Build history of the part. All positions in model axes, mm. A direction names the side the tool comes from. Round coordinates to 2 decimals unless told otherwise and drop trailing zeros. Order: outer loops, then holes, each group sorted by start corner. A loop starts at its lowest first (then second) coordinate and runs counter-clockwise, first axis right, second up. Notation, with made-up numbers: (64, 26) -> (89, 26) arc R20 cw to (89, 42) -> close; hole circle Ø11 at (-11.5, 87.5). An arc over 180 degrees is marked (long way). Answer as CSV lines item,"result". Start each with the question number.
```python
from build123d import *

# Parameters (mm, degrees)
BOSS_EXTRUDE1_DEPTH      = 7.5
SKETCH4_W                = 20
SKETCH4_H                = 3
BOSS_EXTRUDE2_DEPTH      = 35
SKETCH6_W                = 20
SKETCH6_H                = 3
BOSS_EXTRUDE3_DEPTH      = 59.4
SKETCH5_R                = 1.678965669
SKETCH5_R_2              = 1.417070449
SKETCH5_R_3              = 1.591812116
SKETCH5_R_4              = 1.461089302
CUT_EXTRUDE1_DEPTH       = 132.345384388
SKETCH7_R                = 1.6
CUT_EXTRUDE2_DEPTH       = 132.345384388
SKETCH10_W               = 33
SKETCH10_H               = 3
BOSS_EXTRUDE4_DEPTH      = 10
SKETCH11_W               = 8
SKETCH11_H               = 7.5
CUT_EXTRUDE4_DEPTH       = 133.017460966
SKETCH12_W               = 10
SKETCH12_H               = 3
BOSS_EXTRUDE5_DEPTH      = 10
CHAMFER1_SIZE            = 10
CHAMFER1_OF_MIRROR6_SIZE = 10
MIRROR7_START            = -40.25
MIRROR7_DEPTH            = 3
MIRROR7_START_2          = 2.25
MIRROR7_2_DEPTH          = 3
CUT_EXTRUDE5_DEPTH       = 132.345384388


# Read off the part's stored shape, not the designer's step: Mirror7
with BuildPart() as part:
    # Sketch3 → Boss-Extrude1 (new body)
    with BuildSketch(Plane.XY):
        Polygon((0, 0), (19.5, 0), (19.5, 28), (58.5, 28), (58.5, 0), (78, 0), (78, -3), (55.5, -3), (55.5, 25), (22.5, 25), (22.5, -3), (0, -3), align=None)
    boss_extrude1 = extrude(amount=BOSS_EXTRUDE1_DEPTH)

    # Sketch4 → Boss-Extrude2 (add)
    with BuildSketch(Plane(origin=(0, 0, 0), x_dir=(-1, 0, 0), z_dir=(0, 0, -1))):
        with Locations((-39, 26.5)):
            Rectangle(SKETCH4_W, SKETCH4_H)
    extrude(amount=BOSS_EXTRUDE2_DEPTH)

    # Mirror1: Boss-Extrude1 across plane
    add(boss_extrude1.mirror(Plane(origin=(0, 0, -17.5), x_dir=(1, 0, 0), z_dir=(0, 0, -1))))

    # Sketch6 → Boss-Extrude3 (add)
    with BuildSketch(Plane(origin=(0, 0, -42.5), x_dir=(-1, 0, 0), z_dir=(0, 0, -1))):
        with Locations((-39, 26.5)):
            Rectangle(SKETCH6_W, SKETCH6_H)
    extrude(amount=BOSS_EXTRUDE3_DEPTH)

    # Sketch5 → Cut-Extrude1 (cut, through all)
    with BuildSketch(Plane(origin=(0, 0, 0), x_dir=(1, 0, 0), z_dir=(0, 1, 0))):
        with Locations(Location((74, -3.75, 0), (0, 0, 270))):
            Circle(SKETCH5_R)
        with Locations(Location((4, -3.75, 0), (0, 0, 270))):
            Circle(SKETCH5_R_2)
        with Locations(Location((4, 38.75, 0), (0, 0, 270))):
            Circle(SKETCH5_R_3)
        with Locations(Location((74, 38.75, 0), (0, 0, 270))):
            Circle(SKETCH5_R_4)
    extrude(amount=-CUT_EXTRUDE1_DEPTH, mode=Mode.SUBTRACT)

    # Mirror5: Boss-Extrude1 across plane
    add(boss_extrude1.mirror(Plane(origin=(0, 0, -47.2), x_dir=(1, 0, 0), z_dir=(0, 0, -1))))

    # Sketch7 → Cut-Extrude2 (cut, through all)
    with BuildSketch(Plane(origin=(0, 0, 0), x_dir=(1, 0, 0), z_dir=(0, 1, 0))):
        with Locations(Location((64.4, 98.15, 0), (0, 0, 270))):
            Circle(SKETCH7_R)
        with Locations(Location((13.6, 98.15, 0), (0, 0, 270))):
            Circle(SKETCH7_R)
    extrude(amount=-CUT_EXTRUDE2_DEPTH, mode=Mode.SUBTRACT)

    # Sketch10 → Boss-Extrude4 (add)
    with BuildSketch(Plane.XZ.offset(-25)):
        with Locations((39, 6)):
            Rectangle(SKETCH10_W, SKETCH10_H)
    extrude(amount=BOSS_EXTRUDE4_DEPTH)

    # Sketch11 → Cut-Extrude4 (cut, through all)
    with BuildSketch(Plane.XZ.offset(3)):
        with Locations((4, -98.15)):
            Rectangle(SKETCH11_W, SKETCH11_H)
        with Locations((74, -98.15)):
            Rectangle(SKETCH11_W, SKETCH11_H)
    extrude(amount=-CUT_EXTRUDE4_DEPTH, mode=Mode.SUBTRACT)

    # Sketch12 → Boss-Extrude5 (add)
    with BuildSketch(Plane(origin=(0, 0, 0), x_dir=(1, 0, 0), z_dir=(0, 1, 0))):
        with Locations((14.5, 38.75)):
            Rectangle(SKETCH12_W, SKETCH12_H)
    boss_extrude5 = extrude(amount=BOSS_EXTRUDE5_DEPTH)

    # Chamfer1
    chamfer1_edges = [part.edges().sort_by_distance(p)[0] for p in [
        (9.5, 10, -38.75),
    ]]
    chamfer(chamfer1_edges, length=CHAMFER1_SIZE - 0.0001)  # a hair under: the kernel refuses the full size

    # Mirror6: Boss-Extrude5 across plane
    add(boss_extrude5.mirror(Plane.XY.offset(-17.5)))

    # Chamfer1 of Mirror6
    chamfer1_of_mirror6_edges = [part.edges().sort_by_distance(p)[0] for p in [
        (9.5, 10, 3.75),
    ]]
    chamfer(chamfer1_of_mirror6_edges, length=CHAMFER1_OF_MIRROR6_SIZE - 0.0001)  # a hair under: the kernel refuses the full size

    # Mirror7 outline → Mirror7 (add)
    with BuildSketch(Plane.XY.offset(MIRROR7_START)):
        Polygon((58.5, 0), (68.5, 0), (58.5, 10), align=None)
    extrude(amount=MIRROR7_DEPTH)

    # Mirror7 2 outline → Mirror7 2 (add)
    with BuildSketch(Plane.XY.offset(MIRROR7_START_2)):
        Polygon((58.5, 0), (68.5, 0), (58.5, 10), align=None)
    extrude(amount=MIRROR7_2_DEPTH)

    # Sketch13 → Cut-Extrude5 (cut, through all)
    with BuildSketch(Plane.XZ.offset(-25)):
        with BuildLine():
            Line((43, -5.187147638), (43, -27.972265557))
            ThreePointArc((43, -27.972265557), (39, -31.972265557), (35, -27.972265557))
            Line((35, -27.972265557), (35, -5.187147638))
            ThreePointArc((35, -5.187147638), (39, -1.187147638), (43, -5.187147638))
        make_face()
        with BuildLine():
            Line((43, -52.417226503), (43, -84.557823303))
            ThreePointArc((43, -84.557823303), (39, -88.557823303), (35, -84.557823303))
            Line((35, -84.557823303), (35, -52.417226503))
            ThreePointArc((35, -52.417226503), (39, -48.417226503), (43, -52.417226503))
        make_face()
    extrude(amount=-CUT_EXTRUDE5_DEPTH, mode=Mode.SUBTRACT)


solid = part.part
```
Q1. Slice it at B-B, the plane z = -18. Write the cut outline in (x, y).
Q2. Which spindle directions (+Z, -Z, +X, -X, +Y, -Y) get a long thin tool onto all of the face, cutting with end or side? Do faces 4 (the face through (58, 9, -42.5)), 5 (the face through (7, 0, 4)), 6 (the face through (16, 4, -40.25)), 7 (the face through (35, 26, -17)). Say none if no direction does.
Q3. Probe L1, parallel to Z at x = 20.5, y = 2; L2, parallel to X at y = -0.8, z = 3.75; L3, parallel to Z at x = 74, y = -1.3. List the from-to ranges inside material, lowest first.
Q4. Slice it at C-C, the plane x = 64.4. Write the cut outline in (y, z).
Q5. Slice it at A-A, the plane y = 11.5. Write the cut outline in (x, z), plus the area to 3 significant figures.
Q6. Two-plate mould, pull along Z, no slides. Class faces 1 (the face through (61, 3, 2.25)), 2 (the face through (11, -3, 4)), 3 (the face through (61, 3, 5.25)): +Z half, -Z half, draft (parallel to the pull), parting line (faces both ways), or undercut.
Q7. Slice it at D-D, the plane y = 20. Write the cut outline in (x, z), plus the area to 3 significant figures.
Q8. Flat gauge pins, fed straight in: pin 1 Ø5 at (x, y) = (65, 5) entering from -Z; pin 2 Ø2 at (x, z) = (43.5, -57.5) entering from -Y; pin 3 Ø2 at (x, z) = (5.5, -37.5) entering from +Y; pin 4 Ø12 at (x, z) = (39, -70) entering from +Y. Where does each tip first touch, or does it go through?
Solutions:
1,outline,"(29, 25) -> (35, 25) -> (35, 28) -> (29, 28) -> close; (43, 25) -> (49, 25) -> (49, 28) -> (43, 28) -> close"
2,face 4,"+X, +Y, -Y"
2,face 5,"-X, +Y"
2,face 6,"-Z, -X, +Y"
2,face 7,"+Y, -Y"
3,L1,"z = -101.9 to -94.4, -42.5 to -35, 0 to 7.5"
3,L2,"x = 0 to 2.58, 5.42 to 22.5, 55.5 to 72.32, 75.68 to 78"
3,L3,"z = -42.5 to -40.21, -37.29 to -35, 0 to 2.07, 5.43 to 7.5"
4,outline,"(-3, -101.9) -> (0, -101.9) -> (0, -99.75) -> (-3, -99.75) -> close; (-3, -96.55) -> (0, -96.55) -> (0, -94.4) -> (-3, -94.4) -> close; (-3, -42.5) -> (0, -42.5) -> (0, -40.25) -> (4.1, -40.25) -> (4.1, -37.25) -> (0, -37.25) -> (0, -35) -> (-3, -35) -> close; (-3, 0) -> (0, 0) -> (0, 2.25) -> (4.1, 2.25) -> (4.1, 5.25) -> (0, 5.25) -> (0, 7.5) -> (-3, 7.5) -> close"
5,outline,"(19.5, -101.9) -> (22.5, -101.9) -> (22.5, -94.4) -> (19.5, -94.4) -> close; (19.5, -42.5) -> (22.5, -42.5) -> (22.5, -35) -> (19.5, -35) -> close; (19.5, 0) -> (22.5, 0) -> (22.5, 7.5) -> (19.5, 7.5) -> close; (55.5, -101.9) -> (58.5, -101.9) -> (58.5, -94.4) -> (55.5, -94.4) -> close; (55.5, -42.5) -> (58.5, -42.5) -> (58.5, -35) -> (55.5, -35) -> close; (55.5, 0) -> (58.5, 0) -> (58.5, 7.5) -> (55.5, 7.5) -> close"
5,area,"135 mm2"
6,face 1,"undercut"
6,face 2,"draft"
6,face 3,"+Z half"
7,outline,"(19.5, -101.9) -> (22.5, -101.9) -> (22.5, -94.4) -> (19.5, -94.4) -> close; (19.5, -42.5) -> (22.5, -42.5) -> (22.5, -35) -> (19.5, -35) -> close; (19.5, 0) -> (22.5, 0) -> (22.5, 4.5) -> (55.5, 4.5) -> (55.5, 0) -> (58.5, 0) -> (58.5, 7.5) -> (19.5, 7.5) -> close; (55.5, -101.9) -> (58.5, -101.9) -> (58.5, -94.4) -> (55.5, -94.4) -> close; (55.5, -42.5) -> (58.5, -42.5) -> (58.5, -35) -> (55.5, -35) -> close"
7,area,"234 mm2"
8,pin 1,"stops at z = -40.25"
8,pin 2,"stops at y = 25"
8,pin 3,"stops at y = 0"
8,pin 4,"stops at y = 28"
